CAD build for the part. Positions are in the model's coordinates, mm. Coordinates: 2 decimals unless noted, no trailing zeros. Loops run counter-clockwise (first coordinate to the right, second up) from the corner with the lowest first, then second, coordinate; pieces in that order, holes last.
1) Wall check: line 1 along Y through (x, z) = (-13, 0.5) (3 decimals); line 2 along X through (y, z) = (1.5, 0.2) (1 decimal); line 3 along X through (y, z) = (6.5, 0.1) (3 decimals). Give the ranges that are in metal, low to high.
2) Saw through at D-D, the plane y = 6.25. Write the cut outline in (x, z) (3 decimals).
3) Saw through at A-A, the plane x = -12.7. Write the cut outline in (y, z) (3 decimals), and give its area (3 significant figures).
4) Saw through at B-B, the plane y = 0. Write the cut outline in (x, z) (3 decimals), and give its area (3 significant figures).
5) Saw through at C-C, the plane z = 0.5. Write the cut outline in (x, y) (1 decimal).
6) Pin check, flat tip, straight feed: pin 1 Ø3 at (x, y) = (15.875, 0) entering from -Z. Stop position of the tip, or through.
```python
from build123d import *

# Parameters (mm, degrees)
SKETCH1_W           = 44.45
SKETCH1_H           = 19.05
BOSS_EXTRUDE1_DEPTH = 2.54
CUT_EXTRUDE1_REACH  = 26.313
SKETCH2_R           = 4.365625
SKETCH2_R_2         = 1.5875
SKETCH2_R_3         = 2.4892


with BuildPart() as part:
    # Sketch1 → Boss-Extrude1 (new body)
    with BuildSketch(Plane.XY):
        Rectangle(SKETCH1_W, SKETCH1_H)
    extrude(amount=BOSS_EXTRUDE1_DEPTH)

    # Sketch2 → Cut-Extrude1 (cut, up to next)
    with BuildSketch(Plane.XY.offset(2.54), mode=Mode.PRIVATE) as cut_extrude1_sk1:
        with Locations((-12.7, 3.175)):
            Circle(SKETCH2_R)
    cut_extrude1_tool1 = extrude(cut_extrude1_sk1.sketch, amount=-CUT_EXTRUDE1_REACH, mode=Mode.PRIVATE) & part.part
    # Sketch2 → Cut-Extrude1 (cut, up to next)
    with BuildSketch(Plane.XY.offset(2.54), mode=Mode.PRIVATE) as cut_extrude1_sk2:
        with Locations((-1.905, 3.175)):
            Circle(SKETCH2_R_2)
    cut_extrude1_tool2 = extrude(cut_extrude1_sk2.sketch, amount=-CUT_EXTRUDE1_REACH, mode=Mode.PRIVATE) & part.part
    # Sketch2 → Cut-Extrude1 (cut, up to next)
    with BuildSketch(Plane.XY.offset(2.54), mode=Mode.PRIVATE) as cut_extrude1_sk3:
        with Locations((15.875, 0)):
            Circle(SKETCH2_R_3)
    cut_extrude1_tool3 = extrude(cut_extrude1_sk3.sketch, amount=-CUT_EXTRUDE1_REACH, mode=Mode.PRIVATE) & part.part
    add(cut_extrude1_tool1.solids().sort_by_distance((-12.7, 3.175, 2.54))[0], mode=Mode.SUBTRACT)
    add(cut_extrude1_tool2.solids().sort_by_distance((-1.905, 3.175, 2.54))[0], mode=Mode.SUBTRACT)
    add(cut_extrude1_tool3.solids().sort_by_distance((15.875, 0, 2.54))[0], mode=Mode.SUBTRACT)


solid = part.part
```
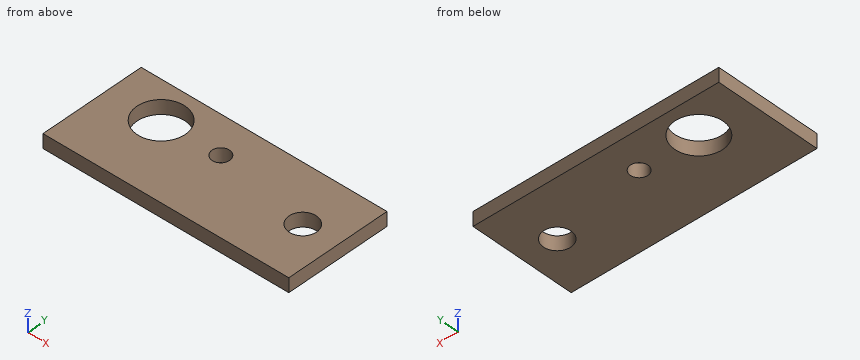
Data:
1. line 1: y = -9.525 to -1.18, 7.53 to 9.525
1. line 2: x = -22.2 to -16.7, -8.7 to 13.9, 17.9 to 22.2
1. line 3: x = -22.225 to -15.529, -9.871 to 22.225
2. outline: (-22.225, 0) - (-15.799, 0) - (-15.799, 2.54) - (-22.225, 2.54) - close; (-9.601, 0) - (22.225, 0) - (22.225, 2.54) - (-9.601, 2.54) - close
3. outline: (-9.525, 0) - (-1.191, 0) - (-1.191, 2.54) - (-9.525, 2.54) - close; (7.541, 0) - (9.525, 0) - (9.525, 2.54) - (7.541, 2.54) - close
3. area: 26.2 mm2
4. outline: (-22.225, 0) - (-15.696, 0) - (-15.696, 2.54) - (-22.225, 2.54) - close; (-9.704, 0) - (13.386, 0) - (13.386, 2.54) - (-9.704, 2.54) - close; (18.364, 0) - (22.225, 0) - (22.225, 2.54) - (18.364, 2.54) - close
4. area: 85.0 mm2
5. outline: (-22.2, -9.5) - (22.2, -9.5) - (22.2, 9.5) - (-22.2, 9.5) - close; hole circle Ø8.7 at (-12.7, 3.2); hole circle Ø3.2 at (-1.9, 3.2); hole circle Ø5 at (15.9, 0)
6. pin 1: passes through
